Check sheet for the modelled part. Datum: model origin and axes. Units: mm. Face numbers are marked on the shaded views. A direction names the side the tool comes from. Coordinates: 2 decimals unless noted, no trailing zeros. Order: outer loops, then holes, each group sorted by start corner. A loop starts at its lowest first (then second) coordinate and runs counter-clockwise, first axis right, second up. Notation, with made-up numbers: (58.25, -25) -> (78.25, -25) arc R24 cw to (78.25, -10) -> close; hole circle Ø8 at (-17, 83). An arc over 180 degrees is marked (long way). Put each result on its own line as item: value. Start each with the question number.
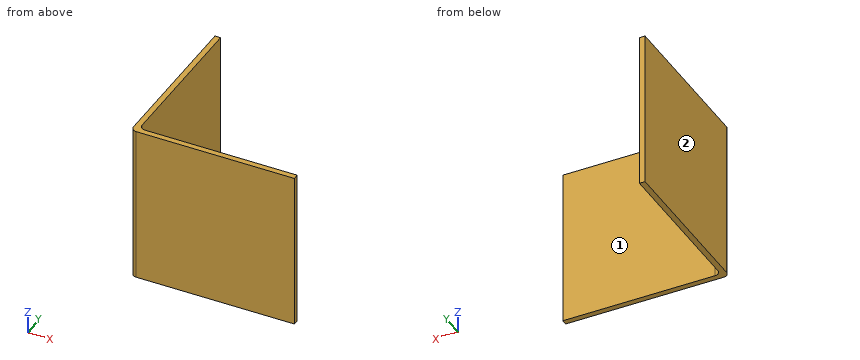
```python
from build123d import *

# Parameters (mm, degrees)
EXTRUDE_1_DEPTH = 28
FILLET_1_R      = 1


with BuildPart() as part:
    # 草图1 → 拉伸-薄壁1 (new body)
    with BuildSketch(Plane.XY):
        Polygon((0, 28), (0, 0), (28, 0), (28, -1), (-1, -1), (-1, 28), align=None)
    extrude(amount=EXTRUDE_1_DEPTH)

    # 圆角1
    fillet_1_edges = [part.edges().sort_by_distance(p)[0] for p in [
        (-1, -1, 14),
        (0, 0, 14),
    ]]
    fillet(fillet_1_edges, radius=FILLET_1_R)


solid = part.part
```
1) Sectioned sample at A-A (z = 5.5). Record the boundary of the cut face in (x, y), plus the area to 3 significant figures.
2) Access from +Z, -Z, +X, -X, +Y, -Y to the whole of each face (thin tool, end or side, straight path). Record for the marked faces 1 and 2.
3) Gauge pin test, flat ends, axial feed: pin 1 (6 mm diameter, centred on y = 13.5, z = 4.5, fed in from +X); pin 2 (13.5 mm diameter, centred on x = 16, z = 17, fed in from +Y). Record the tip position at first contact, or that the pin passes through.
4) Scan lines: line 1 along Y through (x, z) = (5, 16.5); line 2 along Y through (x, z) = (0.5, 13.5). Record each from-to range of solid material in increasing order. Write a range as [from, to].
5) Sectioned sample at B-B (x = 26.25). Record the boundary of the cut face in (y, z).
Entries:
1. outline: (-1, 0) arc R1 ccw to (0, -1) -> (28, -1) -> (28, 0) -> (1, 0) arc R1 cw to (0, 1) -> (0, 28) -> (-1, 28) -> close
1. area: 57.0 mm2
2. face 1: +Z, -Z, +X, +Y
2. face 2: +Z, -Z, -X, +Y, -Y
3. pin 1: stops at x = 0
3. pin 2: stops at y = 0
4. line 1: y = [-1, 0]
4. line 2: y = [-1, 0.13]
5. outline: (-1, 0) -> (0, 0) -> (0, 28) -> (-1, 28) -> close
